For this review, use the dimensioned drawing (mm, ordinates from the lowest corner) and the shaded views. Coordinates: 2 decimals unless noted, no trailing zeros. Write each loop counter-clockwise with the first axis right and the second up, starting at its lowest first coordinate (ties: lowest second). Pieces come first, ordered by that corner, then holes. Notation, with made-up numbers: M -10,56 L 2,56 A25 cw 2,69 Z; hole C 71,10.25 d2. An arc over 180 degrees is marked long. One line per question, with ' | ' between items.
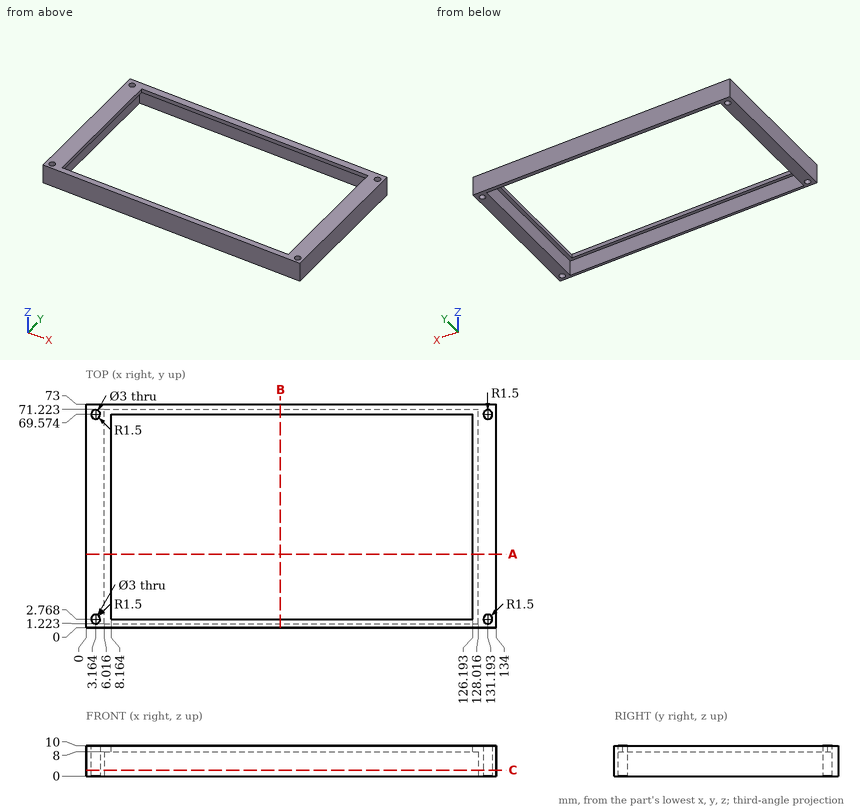
1. Take a section at B-B (x = 63.5). Write out the cut boundary in (y, z).
Answer sheet:
outline: M 0,0 L 1.22,0 L 1.22,8 L 2.77,8 L 2.77,10 L 0,10 Z; M 69.57,8 L 71.22,8 L 71.22,0 L 73,0 L 73,10 L 69.57,10 Z
2. Insertion check: pin 1 Ø1.8 at (x, y) = (3.16, 69.57) entering from -Z. The pin has a flat end and moves straight along its axis. Give the tip position at first contact, or say it passes through.
Answer sheet:
pin 1: through
3. Take a section at A-A (y = 24). Write out the cut boundary in (x, z).
Answer sheet:
outline: M 0,0 L 6.02,0 L 6.02,8 L 8.16,8 L 8.16,10 L 0,10 Z; M 126.19,8 L 128.02,8 L 128.02,0 L 134,0 L 134,10 L 126.19,10 Z
4. To check wall thickness, follow line 1 along X through (y, z) = (49, 5.5); line 2 along Y through (x, z) = (79.5, 9.75); line 3 along Y through (x, z) = (89.5, 7.5). State the ranges of each line that lie inside material, in increasing order. Write a range as [from, to].
Answer sheet:
line 1: [0, 6.02], [128.02, 134] | line 2: [0, 2.77], [69.57, 73] | line 3: [0, 1.22], [71.22, 73]
5. Take a section at C-C (z = 2). Write out the cut boundary in (x, y), then the cut area to 3 significant figures.
Answer sheet:
outline: M 0,0 L 134,0 L 134,73 L 0,73 Z; hole C 3.16,2.77 d3; hole C 3.16,69.57 d3; hole M 6.02,1.22 L 128.02,1.22 L 128.02,71.22 L 6.02,71.22 Z; hole C 131.19,2.77 d3; hole C 131.19,69.57 d3 | area: 1,210 mm^2
